```python
from build123d import *

# Parameters (mm, degrees)
CYLINDER012_R             = 5.1
CYLINDER012_DEPTH         = 50
CYLINDER007_R             = 7.5
CYLINDER007_DEPTH         = 70
CYLINDER009_R             = 6.5
CYLINDER009_DEPTH         = 70
CYLINDER010_R             = 7.5
CYLINDER010_DEPTH         = 70
CYLINDER011_R             = 6.5
CYLINDER011_DEPTH         = 70
FUSION007_PLACEMENT_ANGLE = 180
CYLINDER008_R             = 5.1
CYLINDER008_DEPTH         = 70
BOX003_W                  = 57
BOX003_H                  = 59
BOX003_DEPTH              = 20
CYLINDER004_R             = 6.35
CYLINDER004_DEPTH         = 50
BOX_W                     = 40
BOX_H                     = 20
BOX_DEPTH                 = 30
BOX_PLACEMENT_ANGLE       = 15
CYLINDER001_R             = 5
CYLINDER001_DEPTH         = 50
CYLINDER006_R             = 6.35
CYLINDER006_DEPTH         = 50
BOX001_W                  = 40
BOX001_H                  = 20
BOX001_DEPTH              = 30
BOX001_PLACEMENT_ANGLE    = 15
CYLINDER005_R             = 5
CYLINDER005_DEPTH         = 50
FUSION003_PLACEMENT_ANGLE = 180
BOX002_W                  = 24
BOX002_H                  = 39
BOX002_DEPTH              = 10


with BuildPart() as obj1:
    # Cylinder012 → Cylinder012 (new body)
    with BuildSketch(Plane(origin=(0, -12.5, -17), x_dir=(1, 0, 0), z_dir=(0, 0, 1))):
        Circle(CYLINDER012_R)
    extrude(amount=CYLINDER012_DEPTH)


with BuildPart() as obj2:
    # Cylinder007 → Cylinder007 (new body)
    with BuildSketch(Plane.XY):
        Circle(CYLINDER007_R)
    extrude(amount=CYLINDER007_DEPTH)


with BuildPart() as fusion006:
    # Cylinder009 → Cylinder009 (new body)
    with BuildSketch(Plane(origin=(0, 6.5, 0), x_dir=(1, 0, 0), z_dir=(0, 0, 1))):
        Circle(CYLINDER009_R)
    extrude(amount=CYLINDER009_DEPTH)

    # Fusion006: union obj2
    add(obj2.part)


with BuildPart() as obj3:
    # Cylinder010 → Cylinder010 (new body)
    with BuildSketch(Plane.XY):
        Circle(CYLINDER010_R)
    extrude(amount=CYLINDER010_DEPTH)


with BuildPart() as fusion008:
    # Cylinder011 → Cylinder011 (new body)
    with BuildSketch(Plane(origin=(0, 6.5, 0), x_dir=(1, 0, 0), z_dir=(0, 0, 1))):
        Circle(CYLINDER011_R)
    extrude(amount=CYLINDER011_DEPTH)

    # Fusion007: union obj3
    add(obj3.part)


with BuildPart() as fusion008_1:
    # Fusion007 placement: moved
    add(fusion008.part.rotate(Axis((0, 0, 0), (0, 0, 1)), FUSION007_PLACEMENT_ANGLE))

    # Fusion008: union Fusion006
    add(fusion006.part)


with BuildPart() as cylinder008:
    # Cylinder008 → Cylinder008 (new body)
    with BuildSketch(Plane(origin=(0, 12.5, 0), x_dir=(1, 0, 0), z_dir=(0, 0, 1))):
        Circle(CYLINDER008_R)
    extrude(amount=CYLINDER008_DEPTH)


with BuildPart() as cube003:
    # Box003 → Box003 (new body)
    with BuildSketch(Plane(origin=(-29.5, -29, 51.5), x_dir=(1, 0, 0), z_dir=(0, 0, 1))):
        with Locations((28.5, 29.5)):
            Rectangle(BOX003_W, BOX003_H)
    extrude(amount=BOX003_DEPTH)


with BuildPart() as obj4:
    # Cylinder004 → Cylinder004 (new body)
    with BuildSketch(Plane.XY):
        Circle(CYLINDER004_R)
    extrude(amount=CYLINDER004_DEPTH)


with BuildPart() as cube:
    # Box → Box (new body)
    with BuildSketch(Plane.XY):
        with Locations((20, 10)):
            Rectangle(BOX_W, BOX_H)
    extrude(amount=BOX_DEPTH)


with BuildPart() as cube_1:
    # Box placement: moved
    add(cube.part.moved(Location((-19.558238, 7, 39.759763))).rotate(Axis((-19.558238, 7, 39.759763), (0, 1, 0)), BOX_PLACEMENT_ANGLE))


with BuildPart() as fusion001:
    # Cylinder001 → Cylinder001 (new body)
    with BuildSketch(Plane(origin=(0, 12.5, 0), x_dir=(1, 0, 0), z_dir=(0, 0, 1))):
        Circle(CYLINDER001_R)
    extrude(amount=CYLINDER001_DEPTH)

    # Fusion: union Cube
    add(cube_1.part)

    # Fusion001: union obj4
    add(obj4.part)


with BuildPart() as obj5:
    # Cylinder006 → Cylinder006 (new body)
    with BuildSketch(Plane.XY):
        Circle(CYLINDER006_R)
    extrude(amount=CYLINDER006_DEPTH)


with BuildPart() as cube001:
    # Box001 → Box001 (new body)
    with BuildSketch(Plane.XY):
        with Locations((20, 10)):
            Rectangle(BOX001_W, BOX001_H)
    extrude(amount=BOX001_DEPTH)


with BuildPart() as cube001_1:
    # Box001 placement: moved
    add(cube001.part.moved(Location((-19.558238, 7, 39.759763))).rotate(Axis((-19.558238, 7, 39.759763), (0, 1, 0)), BOX001_PLACEMENT_ANGLE))


with BuildPart() as fusion004:
    # Cylinder005 → Cylinder005 (new body)
    with BuildSketch(Plane(origin=(0, 12.5, 0), x_dir=(1, 0, 0), z_dir=(0, 0, 1))):
        Circle(CYLINDER005_R)
    extrude(amount=CYLINDER005_DEPTH)

    # Fusion002: union Cube001
    add(cube001_1.part)

    # Fusion003: union obj5
    add(obj5.part)


with BuildPart() as fusion004_1:
    # Fusion003 placement: moved
    add(fusion004.part.rotate(Axis((0, 0, 0), (0, 0, 1)), FUSION003_PLACEMENT_ANGLE))

    # Fusion004: union Fusion001
    add(fusion001.part)


with BuildPart() as cut003:
    # Box002 → Box002 (new body)
    with BuildSketch(Plane(origin=(-12, -13, 41.5), x_dir=(1, 0, 0), z_dir=(0, 0, 1))):
        with Locations((12, 19.5)):
            Rectangle(BOX002_W, BOX002_H)
    extrude(amount=BOX002_DEPTH)

    # Fusion005: union Fusion004
    add(fusion004_1.part)

    # Cut: cut Cube003
    add(cube003.part, mode=Mode.SUBTRACT)

    # Cut001: cut Cylinder008
    add(cylinder008.part, mode=Mode.SUBTRACT)

    # Cut002: cut Fusion008
    add(fusion008_1.part, mode=Mode.SUBTRACT)

    # Cut003: cut obj1
    add(obj1.part, mode=Mode.SUBTRACT)


solid = cut003.part
```
Can you work these out from the model? Positions are in its coordinate system, mm. A direction names the side the tool comes from. Coordinates: 2 decimals unless noted, no trailing zeros. Loops run counter-clockwise (first coordinate to the right, second up) from the corner with the lowest first, then second, coordinate; pieces in that order, holes last. Notation, with made-up numbers: (25, 73) -> (50, 73) arc R21 cw to (50, 98) -> close; hole circle Ø7 at (78, 40). An arc over 180 degrees is marked (long way). Put each result on its own line as item: value. Start each with the question number.
Q1. If I drill on line 1 (Y direction, x = 0, z = 37); line 2 (X direction, y = -6.5, z = 46.5); line 3 (Y direction, x = -9.5, z = 40), over which ranges is the centre line in solid material (lowest first)? Write a range as [from, to].
Q2. I want a section at A-A (y = -6). Write out the boundary of the cut face in (x, z), plus the area to 3 significant figures.
Q3. I'm going to push flat-ended pins straight in: P1, Ø3, axis at x = -9, y = -2.5, coming from the -Z side; P2, Ø2, axis at x = 2, y = -14.5, coming from the -Z side; P3, Ø5, axis at y = 2, z = 48, coming from the +X side. Where does each tip first touch, or does it pass through?
Q4. I want a section at B-B (x = -2). Write out the boundary of the cut face in (y, z).
Q5. For faces 1 (the face through (-0.51, 19.362, 34.656)), 2 (the face through (6.193, 8.473, 44.09)), 3 (the face through (18.007, -16.86, 45.548)), 4 (the face through (-9, 0, 41.5)), 5 (the face through (-12, 0, 46)), which set-ups out of +Z, -Z, +X, -X, +Y, -Y let a thin tool reach every point of the face, with its end or its side?
Q6. Thinking about a two-plate mould opening in X: for faces 6 (the face through (-6.365, 7.817, 43.546)), 7 (the face through (12, 0, 46)), 8 (the face through (13, -7, 43)), which applies, pulls with the +X half, pulls with the -X half, needs draft (parallel to the pull), parting line crosses it, or undercut?
Q7. I want a section at D-D (z = 44.5). Write out the boundary of the cut face in (x, y).
Q8. I want a section at C-C (z = 37.5). Write out the boundary of the cut face in (x, y), plus the area to 3 significant figures.
Taken from the geometry:
1. line 1: y = [-27, -13], [17.6, 27]
1. line 2: x = [-12, -6.5], [6.5, 12]
1. line 3: y = [-27, -7], [7, 27]
2. outline: (-12, 41.5) -> (-6.48, 41.5) -> (-6.48, 51.5) -> (-12, 51.5) -> close; (6.48, 41.5) -> (12, 41.5) -> (12, 51.5) -> (6.48, 51.5) -> close
2. area: 110 mm2
3. P1: stops at z = 41.5
3. P2: stops at z = 33
3. P3: stops at x = 12
4. outline: (-27, 33.98) -> (-17.08, 33.98) -> (-17.08, 33) -> (-12.68, 33) -> (-12.68, 51.5) -> (-27, 51.5) -> close; (17.19, 35.06) -> (27, 35.06) -> (27, 51.5) -> (17.19, 51.5) -> close
5. face 1: -Z, -X, +Y
5. face 2: +Z, -Z
5. face 3: +Z, +X, -Y
5. face 4: -Z, +X, -X
5. face 5: +Z, -Z, -X
6. face 6: undercut
6. face 7: pulls with the +X half
6. face 8: needs draft
7. outline: (-23.12, -27) -> (18.29, -27) -> (18.29, -7) -> (12, -7) -> (12, 7) -> (23.12, 7) -> (23.12, 27) -> (-18.29, 27) -> (-18.29, 7) -> (-12, 7) -> (-12, -7) -> (-23.12, -7) -> close; hole (-6.13, -4.33) arc R6.5 ccw (long way) to (6.13, -4.33) arc R7.5 ccw to (6.13, 4.33) arc R6.5 ccw to (4.83, 10.85) arc R5.1 ccw (long way) to (-4.83, 10.85) arc R6.5 ccw to (-6.13, 4.33) arc R7.5 ccw to start
8. outline: (-21.25, -27) -> (11.12, -27) -> (11.12, -7) -> (6.48, -7) arc R6.5 cw to (-6.48, -7) -> (-21.25, -7) -> close; (-11.12, 7) -> (-6.48, 7) arc R6.5 cw to (-4.83, 10.85) arc R5.1 cw (long way) to (4.83, 10.85) arc R6.5 cw to (6.48, 7) -> (21.25, 7) -> (21.25, 27) -> (-11.12, 27) -> close
8. area: 1,130 mm2
